from build123d import *

# Parameters (mm, degrees)
SKETCH_2_W             = 27.9
SKETCH_2_H             = 17.9
EXTRUDE_1_DEPTH        = 12.5
HOLE_WIZARD_M3_1_D     = 2.5
HOLE_WIZARD_M3_2_D     = 2.5
HOLE_WIZARD_M3_3_D     = 2.5
SKETCH_9_W             = 19.9
SKETCH_9_H             = 9.9
CUT_EXTRUDE_1_DEPTH    = 26
CHAMFER_2_SIZE         = 0.5
HOLE_WIZARD_M3_4_D     = 2.5
HOLE_WIZARD_M3_6_D     = 2.5
HOLE_WIZARD_M3_6_DEPTH = 4
HOLE_WIZARD_M3_7_D     = 2.5
FILLET_1_R             = 1


with BuildPart() as part:
    # 草图2 → 凸台-拉伸1 (new body, symmetric)
    with BuildSketch(Plane.XY):
        Rectangle(SKETCH_2_W, SKETCH_2_H)
    extrude(amount=EXTRUDE_1_DEPTH, both=True)

    # M3 螺纹孔1 (through all)
    with Locations(Plane(origin=(1, -8.95, -8.5), x_dir=(0, 0, -1), z_dir=(0, -1, 0))):
        with Locations((0, 0)):
            Hole(HOLE_WIZARD_M3_1_D / 2)

    # M3 螺纹孔2 (through all)
    with Locations(Plane(origin=(-13.95, 0, -8.5), x_dir=(0, 0, -1), z_dir=(-1, 0, 0))):
        with Locations((0, 0)):
            Hole(HOLE_WIZARD_M3_2_D / 2)

    # M3 螺纹孔3 (through all)
    with Locations(Plane(origin=(1, -8.95, 6.5), x_dir=(0, 0, -1), z_dir=(0, -1, 0))):
        with Locations((0, 0)):
            Hole(HOLE_WIZARD_M3_3_D / 2)

    # 草图9 → 切除-拉伸1 (cut, through all)
    with BuildSketch(Plane(origin=(0, 0, -12.5), x_dir=(-1, 0, 0), z_dir=(0, 0, -1))):
        Rectangle(SKETCH_9_W, SKETCH_9_H)
    extrude(amount=-CUT_EXTRUDE_1_DEPTH, mode=Mode.SUBTRACT)

    # 倒角2
    chamfer_2_edges = [part.edges().sort_by_distance(p)[0] for p in [
        (-13.95, 0, 12.5),
        (0, -8.95, 12.5),
        (13.95, 0, 12.5),
        (0, -8.95, -12.5),
        (-13.95, 0, -12.5),
        (0, 8.95, -12.5),
        (13.95, 0, -12.5),
        (13.95, -8.95, 0),
        (-13.95, -8.95, 0),
        (-13.95, 8.95, 0),
        (13.95, 8.95, 0),
        (0, 8.95, 12.5),
    ]]
    chamfer(chamfer_2_edges, length=CHAMFER_2_SIZE)

    # M3 螺纹孔4 (through all)
    with Locations(Plane(origin=(13.95, 0, 1.5), x_dir=(0, 0, 1), z_dir=(1, 0, 0))):
        with Locations((0, 0)):
            Hole(HOLE_WIZARD_M3_4_D / 2)

    # M3 螺纹孔6
    with Locations(Plane(origin=(13.95, 0, 6), x_dir=(0, 0, 1), z_dir=(1, 0, 0))):
        with Locations((0, 0)):
            Hole(HOLE_WIZARD_M3_6_D / 2, depth=HOLE_WIZARD_M3_6_DEPTH)

    # M3 螺纹孔7 (through all)
    with Locations(Plane(origin=(1, 8.95, 1), x_dir=(0, 0, 1), z_dir=(0, 1, 0))):
        with Locations((0, 0)):
            Hole(HOLE_WIZARD_M3_7_D / 2)

    # 圆角1
    fillet_1_edges = [part.edges().sort_by_distance(p)[0] for p in [
        (-9.95, 4.95, 0),
        (9.95, -4.95, 0),
        (9.95, 4.95, 0),
        (-9.95, -4.95, 0),
    ]]
    fillet(fillet_1_edges, radius=FILLET_1_R)


solid = part.part
CAD build for the part. Positions are in the model's coordinates, mm. A direction names the side the tool comes from. Coordinates: 2 decimals unless noted, no trailing zeros. Order: outer loops, then holes, each group sorted by start corner. A loop starts at its lowest first (then second) coordinate and runs counter-clockwise, first axis right, second up. Notation, with made-up numbers: (48.5, 44.25) -> (77.5, 44.25) arc R19 ccw to (77.5, 50.25) -> close; hole circle Ø8 at (-31, 62). An arc over 180 degrees is marked (long way). Answer in a Markdown table with one row per item.
1) Band-saw the part on B-B (x = -2). List the corners of the cut face in (y, z), and give its area (4 significant figures).
Check values:
| item | result |
|---|---|
| outline | (-8.95, -12) -> (-8.45, -12.5) -> (-4.95, -12.5) -> (-4.95, 12.5) -> (-8.45, 12.5) -> (-8.95, 12) -> close; (4.95, -12.5) -> (8.45, -12.5) -> (8.95, -12) -> (8.95, 12) -> (8.45, 12.5) -> (4.95, 12.5) -> close |
| area | 199.5 mm2 |
2) Band-saw the part on A-A (z = -8.5). Give the number of separate pieces and of enclosed holes in the cut face, and give its area (3 significant figures).
Check values:
| item | result |
|---|---|
| separate pieces | 4 |
| enclosed holes | 0 |
| area | 263 mm2 |
3) Drill centre lines: line 1 (X direction, y = -6.1, z = 1); line 2 (Y direction, x = -3.5, z = 5); line 3 (X direction, y = 4, z = -4.75). Where is each one in solid material? Low to high.
Check values:
| item | result |
|---|---|
| line 1 | -13.95 to -0.25, 2.25 to 13.95 |
| line 2 | -8.95 to -4.95, 4.95 to 8.95 |
| line 3 | -13.95 to -9.95, 9.95 to 13.95 |
4) Which spindle directions (+Z, -Z, +X, -X, +Y, -Y) get a long thin tool onto all of the face, cutting with end or side? Do faces 1 (the face through (9.95, 0, 0)), 2 (the face through (1.05, 6.98, -9.75)). Say none if no direction does.
Check values:
| item | result |
|---|---|
| face 1 | +Z, -Z |
| face 2 | +Y, -Y |
5) Band-saw the part on C-C (y = -2.25). List the corners of the cut face in (x, z), and give its area (4 significant figures).
Check values:
| item | result |
|---|---|
| outline | (-13.95, -12) -> (-13.45, -12.5) -> (-9.95, -12.5) -> (-9.95, 12.5) -> (-13.45, 12.5) -> (-13.95, 12) -> close; (9.95, -12.5) -> (13.45, -12.5) -> (13.95, -12) -> (13.95, 12) -> (13.45, 12.5) -> (9.95, 12.5) -> close |
| area | 199.5 mm2 |
6) Mould opens along X. For faces 3 (the face through (11.92, -0.05, 7.25)), 4 (the face through (13.95, 0, 0)), 5 (the face through (9.649, -4.665, 0.175)) say: pulls with the +X half, pulls with the -X half, needs draft (parallel to the pull), parting line crosses it, or undercut.
Check values:
| item | result |
|---|---|
| face 3 | needs draft |
| face 4 | pulls with the +X half |
| face 5 | undercut |
